Read the model definition and answer for the solid it produces. Units are mm, in the model's axes. A direction names the side the tool comes from. Coordinates: 2 decimals unless noted, no trailing zeros. Write each loop counter-clockwise with the first axis right and the second up, starting at its lowest first coordinate (ties: lowest second). Pieces come first, ordered by that corner, then holes. Notation, with made-up numbers: (-2.5, 47.5) -> (18.5, 47.5) arc R32 cw to (18.5, 85.5) -> close; hole circle Ø8 at (58.25, 7.25). An arc over 180 degrees is marked (long way). One line per item, written item: value. Start each with the question number.
from build123d import *

# Parameters (mm, degrees)
F1_DEPTH = 25.4


with BuildPart() as f1:
    # F0 (on Right) → F1 (new body)
    with BuildSketch(Plane.YZ):
        with BuildLine():
            Line((16.450379, 12.7), (-38.1, 12.7))
            Line((-38.1, 12.7), (-38.1, -12.7))
            Line((-38.1, -12.7), (16.450379, -12.7))
            Line((16.450379, -12.7), (38.1, -12.7))
            Line((38.1, -12.7), (38.1, -10.063089))
            ThreePointArc((38.1, -10.063089), (37.914013, -9.614076), (37.465, -9.428089))
            Line((37.465, -9.428089), (17.518706, -9.428089))
            ThreePointArc((17.518706, -9.428089), (13.028578, -7.568217), (11.168706, -3.078089))
            Line((11.168706, -3.078089), (11.168706, 3.078089))
            ThreePointArc((11.168706, 3.078089), (13.028578, 7.568217), (17.518706, 9.428089))
            Line((17.518706, 9.428089), (37.465, 9.428089))
            ThreePointArc((37.465, 9.428089), (37.914013, 9.614076), (38.1, 10.063089))
            Line((38.1, 10.063089), (38.1, 12.7))
            Line((38.1, 12.7), (16.450379, 12.7))
        make_face()
        Polygon((16.450379, 16.587621), (16.450379, 12.7), (38.1, 12.7), align=None)
        Polygon((38.1, -12.7), (16.450379, -12.7), (16.450379, -16.587621), align=None)
    extrude(amount=F1_DEPTH)


solid = f1.part
1. A cutting plane is placed at B-B on y = -27. Give the vertices of the cut face in (x, z).
2. Given pin 1 (1.2 mm diameter, centred on x = 10, z = 14.5, fed in from -Y); pin 2 (10 mm diameter, centred on x = 8, y = 32, fed in from +Z); pin 3 (8 mm diameter, centred on x = 3, y = -9.5, fed in from -Z), each flat-ended and moving along its own axis, determine where each tip first touches the part or whether it passes through.
3. For a pull along Z with two mould halves and no side action, classify faces 5 (the face through (12.52, 12.98, 7.52)), 6 (the face through (12.522, 27.427, 14.617)), 7 (the face through (12.52, 27.12, -14.67)) as +Z half, -Z half, draft (parallel to the pull), parting line (faces both ways), or undercut.
4. A cutting plane is placed at A-A on x = 3.75. Give the vertices of the cut face in (y, z) (3 decimals), then the cut area to 3 significant figures.
5. Find the intervals of material crossed by probe 1 along Z at (x, y) = (5.75, -1); probe 2 along Y at (x, z) = (5.5, -3); probe 3 along Z at (x, y) = (12.75, 16.5), in increasing order. Write a range as from..to.
6. A tool of negligible diameter and unlimited length cuts with its end or side. For faces 1 (the face through (13, 16.45, -15)), 2 (the face through (13, 27, 9.428)), 3 (the face through (25.4, -9, 0)), 4 (the face through (13, 16.45, 15)), from which of +Z, -Z, +X, -X, +Y, -Y can it reach the whole face along a straight path? Write none if from no direction.
7. A cutting plane is placed at C-C on z = -2. Give the vertices of the cut face in (x, y), then the cut area to 3 significant figures.
Derived:
1. outline: (0, -12.7) -> (25.4, -12.7) -> (25.4, 12.7) -> (0, 12.7) -> close
2. pin 1: stops at y = 16.45
2. pin 2: stops at z = 14.69
2. pin 3: stops at z = -12.7
3. face 5: undercut
3. face 6: +Z half
3. face 7: -Z half
4. outline: (-38.1, -12.7) -> (16.45, -12.7) -> (16.45, -16.588) -> (38.1, -12.7) -> (38.1, -10.063) arc R0.635 ccw to (37.465, -9.428) -> (17.519, -9.428) arc R6.35 cw to (11.169, -3.078) -> (11.169, 3.078) arc R6.35 cw to (17.519, 9.428) -> (37.465, 9.428) arc R0.635 ccw to (38.1, 10.063) -> (38.1, 12.7) -> (16.45, 16.588) -> (16.45, 12.7) -> (-38.1, 12.7) -> close
4. area: 1,530 mm2
5. probe 1: z = -12.7..12.7
5. probe 2: y = -38.1..11.17
5. probe 3: z = -16.58..-9.35, 9.35..16.58
6. face 1: -Z, +X, -X, -Y
6. face 2: +X, -X, +Y
6. face 3: +Z, -Z, +X, +Y, -Y
6. face 4: +Z, +X, -X, -Y
7. outline: (0, -38.1) -> (25.4, -38.1) -> (25.4, 11.17) -> (0, 11.17) -> close
7. area: 1,250 mm2
